The drawing under review shows one solid part. Ordinate dimensions are in mm from its lowest x, y, z. A direction names the side the tool comes from. Give positions to 0.01 mm unless a question says otherwise; leave off trailing zeros. Loops run counter-clockwise (first coordinate to the right, second up) from the corner with the lowest first, then second, coordinate; pieces in that order, holes last. Notation, with made-up numbers: M 86,67.25 L 130,67.25 A22 cw 130,83.25 Z; hole C -23.75,-29 d11. An arc over 180 degrees is marked long. Write item = value, one per line. Start each with the question number.
1. For pin 1 (12 mm diameter, centred on x = 20, y = 4.5, fed in from +Z); pin 2 (8 mm diameter, centred on y = 8, z = 7.5, fed in from -X); pin 3 (2 mm diameter, centred on y = 30.5, z = 6, fed in from -X); pin 4 (4 mm diameter, centred on x = 13.41, z = 17, fed in from -Y), all flat-tipped, find the tip position at first contact; note any pin that passes through.
2. We need section D-D on y = 5. Give the boundary of the cut face in (x, z).
3. We need section C-C on x = 4.5. Give the boundary of the cut face in (y, z), then the cut area to 3 significant figures.
4. Wall thickness on line 1 along Z through (x, y) = (14.5, 15.5) (1 decimal); line 2 along Y through (x, z) = (13, 5); line 3 along X through (y, z) = (12.5, 17): over which ranges is each line inside the solid? List them lowest first. Write a range as from..to.
5. We need section B-B on y = 9.5. Give the boundary of the cut face in (x, z) (1 decimal), then the cut area to 3 significant figures.
6. Draft analysis for pull direction Z (two halves, no side actions). For the marked faces 4, 5 and 6, state which applies: pulls with the +Z half, pulls with the -Z half, needs draft (parallel to the pull), parting line crosses it, or undercut.
7. For the marked faces 1, 2 and 3, list the 3-axis set-ups (+Z, -Z, +X, -X, +Y, -Y) from which the entire face can be reached by the end or side of a thin tool; tool diameter is ignored.
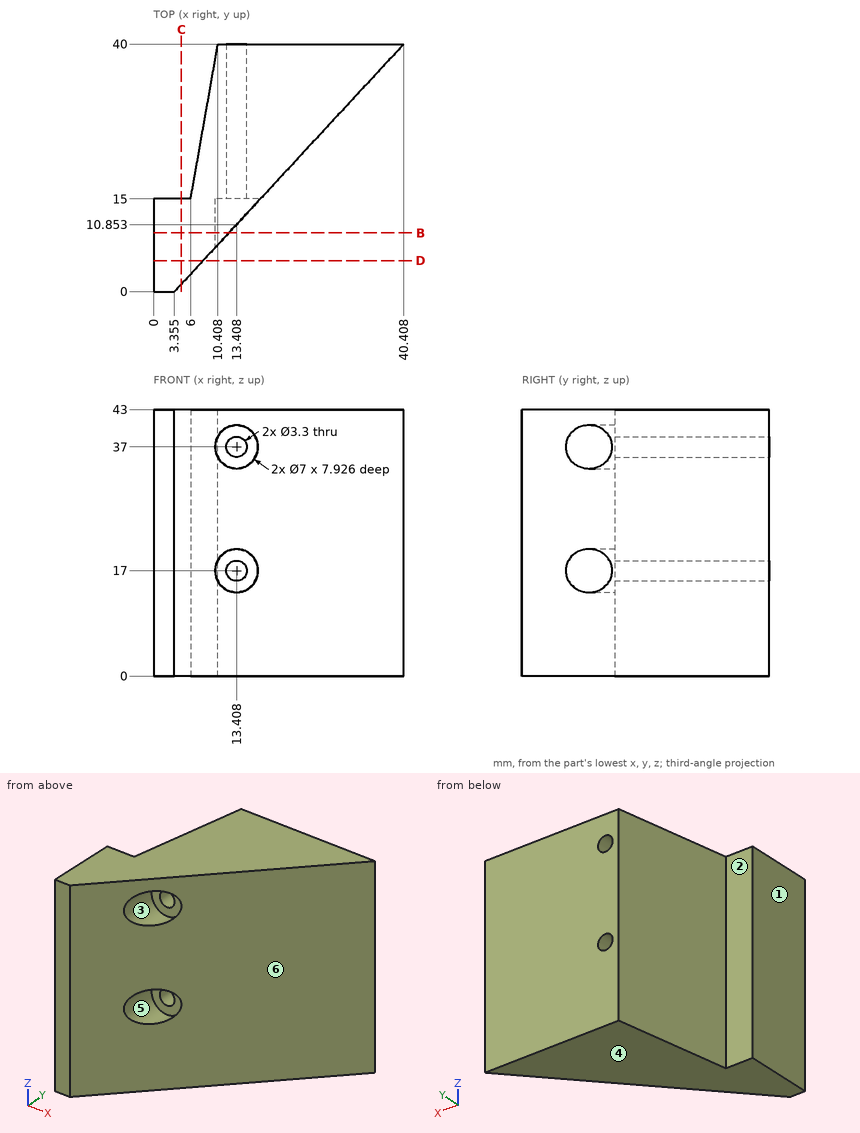
Final values:
q1.pin_1 = through
q1.pin_2 = 0
q1.pin_3 = 8.56
q1.pin_4 = 15
q2.outline = M 0,0 L 7.99,0 L 7.99,43 L 0,43 Z
q3.outline = M 1.24,0 L 15,0 L 15,43 L 1.24,43 Z
q3.area = 592 mm²
q4.line_1 = 0..15.8, 18.2..35.8, 38.2..43
q4.line_2 = 10.41..40
q4.line_3 = 0..9.91
q5.outline = M 0,0 L 12.2,0 L 12.2,13.7 A3.5 cw 12.2,20.3 L 12.2,33.7 A3.5 cw 12.2,40.3 L 12.2,43 L 0,43 Z
q5.area = 501 mm²
q6.face_4 = pulls with the -Z half
q6.face_5 = undercut
q6.face_6 = needs draft
q7.face_1 = +Z, -Z, -X, +Y, -Y
q7.face_2 = +Z, -Z, -X, +Y
q7.face_3 = -Y
